Source: CAD feature listing. Evaluate the final solid. Frame: model axes, mm. Give positions to 0.01 mm unless a question says otherwise; leave off trailing zeros. Write each loop counter-clockwise with the first axis right and the second up, starting at its lowest first coordinate (ties: lowest second). Pieces come first, ordered by that corner, then holes. Notation, with made-up numbers: M -20,62 L 36,62 A29 cw 36,96 Z; hole C 82,-35.5 d7. An arc over 180 degrees is marked long. Return JSON: item names as keys, results as strings.
```python
from build123d import *

# Parameters (mm, degrees)
PARED_Y_1_4IN_START          = 95.25
CROQUIS1_W                   = 228.6
CROQUIS1_H                   = 50.8
PARED_Y_1_4IN_DEPTH          = 6.35
ROSCA_M3_INFERIOR_START      = 12.7
CROQUIS2_R                   = 1.25
ROSCA_M3_INFERIOR_DEPTH      = 10
ROSCA_M3_SUPERIOR_START      = 53.5
CROQUIS3_R                   = 1.25
ROSCA_M3_SUPERIOR_DEPTH      = 10
BARRENOS_M3_ESQUINAS_START   = 95.25
CROQUIS4_R                   = 1.7
BARRENOS_M3_ESQUINAS_DEPTH   = 6.35
REFRENTADO_M3_ESQUINAS_START = 98.4
CROQUIS5_R                   = 2.9
REFRENTADO_M3_ESQUINAS_DEPTH = 3.2
RANURAS_VENTILACION_START    = 95.25
RANURAS_VENTILACION_DEPTH    = 6.35


with BuildPart() as part:
    # Croquis1 → Pared_+Y_1-4in (new body)
    with BuildSketch(Plane(origin=(0, 0, 0), x_dir=(1, 0, 0), z_dir=(0, 1, 0)).offset(PARED_Y_1_4IN_START)):
        with Locations((-25.4, -38.1)):
            Rectangle(CROQUIS1_W, CROQUIS1_H)
    extrude(amount=PARED_Y_1_4IN_DEPTH)

    # Croquis2 → Rosca_M3_inferior (cut)
    with BuildSketch(Plane.XY.offset(ROSCA_M3_INFERIOR_START)):
        with Locations((-125, 98.425)):
            Circle(CROQUIS2_R)
        with Locations((-30, 98.425)):
            Circle(CROQUIS2_R)
        with Locations((70, 98.425)):
            Circle(CROQUIS2_R)
    extrude(amount=ROSCA_M3_INFERIOR_DEPTH, mode=Mode.SUBTRACT)

    # Croquis3 → Rosca_M3_superior (cut)
    with BuildSketch(Plane.XY.offset(ROSCA_M3_SUPERIOR_START)):
        with Locations((-125, 98.425)):
            Circle(CROQUIS3_R)
        with Locations((-30, 98.425)):
            Circle(CROQUIS3_R)
        with Locations((70, 98.425)):
            Circle(CROQUIS3_R)
    extrude(amount=ROSCA_M3_SUPERIOR_DEPTH, mode=Mode.SUBTRACT)

    # Croquis4 → Barrenos_M3_esquinas (cut)
    with BuildSketch(Plane(origin=(0, 0, 0), x_dir=(1, 0, 0), z_dir=(0, 1, 0)).offset(BARRENOS_M3_ESQUINAS_START)):
        with Locations(Location((-136.525, -25, 0), (0, 0, 270))):
            Circle(CROQUIS4_R)
        with Locations(Location((-136.525, -50, 0), (0, 0, 270))):
            Circle(CROQUIS4_R)
        with Locations(Location((85.725, -25, 0), (0, 0, 270))):
            Circle(CROQUIS4_R)
        with Locations(Location((85.725, -50, 0), (0, 0, 270))):
            Circle(CROQUIS4_R)
    extrude(amount=BARRENOS_M3_ESQUINAS_DEPTH, mode=Mode.SUBTRACT)

    # Croquis5 → Refrentado_M3_esquinas (cut)
    with BuildSketch(Plane(origin=(0, 0, 0), x_dir=(1, 0, 0), z_dir=(0, 1, 0)).offset(REFRENTADO_M3_ESQUINAS_START)):
        with Locations(Location((-136.525, -25, 0), (0, 0, 270))):
            Circle(CROQUIS5_R)
        with Locations(Location((-136.525, -50, 0), (0, 0, 270))):
            Circle(CROQUIS5_R)
        with Locations(Location((85.725, -25, 0), (0, 0, 270))):
            Circle(CROQUIS5_R)
        with Locations(Location((85.725, -50, 0), (0, 0, 270))):
            Circle(CROQUIS5_R)
    extrude(amount=REFRENTADO_M3_ESQUINAS_DEPTH, mode=Mode.SUBTRACT)

    # Croquis6 → Ranuras_ventilacion (cut)
    with BuildSketch(Plane(origin=(0, 0, 0), x_dir=(1, 0, 0), z_dir=(0, 1, 0)).offset(RANURAS_VENTILACION_START)):
        with BuildLine():
            Line((-107, -24.7), (-107, -51.5))
            ThreePointArc((-107, -51.5), (-110, -54.5), (-113, -51.5))
            Line((-113, -51.5), (-113, -24.7))
            ThreePointArc((-113, -24.7), (-110, -21.7), (-107, -24.7))
        make_face()
        with BuildLine():
            Line((-92, -24.7), (-92, -51.5))
            ThreePointArc((-92, -51.5), (-95, -54.5), (-98, -51.5))
            Line((-98, -51.5), (-98, -24.7))
            ThreePointArc((-98, -24.7), (-95, -21.7), (-92, -24.7))
        make_face()
        with BuildLine():
            Line((-77, -24.7), (-77, -51.5))
            ThreePointArc((-77, -51.5), (-80, -54.5), (-83, -51.5))
            Line((-83, -51.5), (-83, -24.7))
            ThreePointArc((-83, -24.7), (-80, -21.7), (-77, -24.7))
        make_face()
        with BuildLine():
            Line((-62, -24.7), (-62, -51.5))
            ThreePointArc((-62, -51.5), (-65, -54.5), (-68, -51.5))
            Line((-68, -51.5), (-68, -24.7))
            ThreePointArc((-68, -24.7), (-65, -21.7), (-62, -24.7))
        make_face()
        with BuildLine():
            Line((-42, -24.7), (-42, -51.5))
            ThreePointArc((-42, -51.5), (-45, -54.5), (-48, -51.5))
            Line((-48, -51.5), (-48, -24.7))
            ThreePointArc((-48, -24.7), (-45, -21.7), (-42, -24.7))
        make_face()
        with BuildLine():
            Line((-12, -24.7), (-12, -51.5))
            ThreePointArc((-12, -51.5), (-15, -54.5), (-18, -51.5))
            Line((-18, -51.5), (-18, -24.7))
            ThreePointArc((-18, -24.7), (-15, -21.7), (-12, -24.7))
        make_face()
        with BuildLine():
            Line((3, -24.7), (3, -51.5))
            ThreePointArc((3, -51.5), (0, -54.5), (-3, -51.5))
            Line((-3, -51.5), (-3, -24.7))
            ThreePointArc((-3, -24.7), (0, -21.7), (3, -24.7))
        make_face()
        with BuildLine():
            Line((18, -24.7), (18, -51.5))
            ThreePointArc((18, -51.5), (15, -54.5), (12, -51.5))
            Line((12, -51.5), (12, -24.7))
            ThreePointArc((12, -24.7), (15, -21.7), (18, -24.7))
        make_face()
        with BuildLine():
            Line((33, -24.7), (33, -51.5))
            ThreePointArc((33, -51.5), (30, -54.5), (27, -51.5))
            Line((27, -51.5), (27, -24.7))
            ThreePointArc((27, -24.7), (30, -21.7), (33, -24.7))
        make_face()
        with BuildLine():
            Line((48, -24.7), (48, -51.5))
            ThreePointArc((48, -51.5), (45, -54.5), (42, -51.5))
            Line((42, -51.5), (42, -24.7))
            ThreePointArc((42, -24.7), (45, -21.7), (48, -24.7))
        make_face()
        with BuildLine():
            Line((58, -24.7), (58, -51.5))
            ThreePointArc((58, -51.5), (55, -54.5), (52, -51.5))
            Line((52, -51.5), (52, -24.7))
            ThreePointArc((52, -24.7), (55, -21.7), (58, -24.7))
        make_face()
    extrude(amount=RANURAS_VENTILACION_DEPTH, mode=Mode.SUBTRACT)


solid = part.part
```
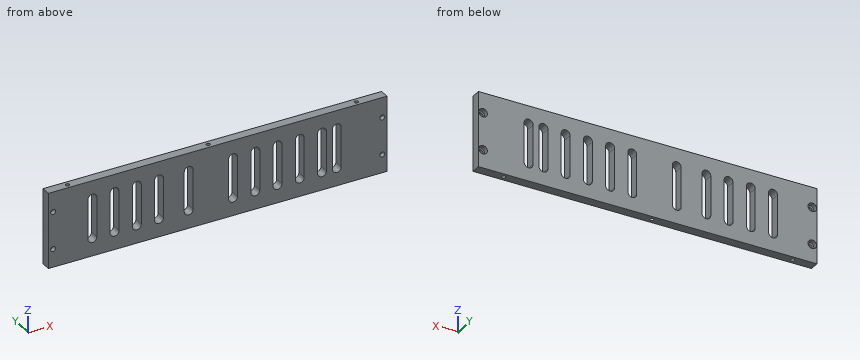
1) Cut plane A-A, the plane x = 0. Return the cut outline in (y, z).
Numbers:
{"outline": "M 95.25,12.7 L 101.6,12.7 L 101.6,21.7 L 95.25,21.7 Z; M 95.25,54.5 L 101.6,54.5 L 101.6,63.5 L 95.25,63.5 Z"}
2) Line query: line 1 (X direction, y = 98.5, z = 15.5); line 2 (Z direction, x = -78, y = 97.75); line 3 (Z direction, x = -64, y = 99.25). Output: solid intervals per line, ascending. Write a range as [from, to].
Numbers:
{"line 1": "x = [-139.7, -126.25], [-123.75, -31.25], [-28.75, 68.75], [71.25, 88.9]", "line 2": "z = [12.7, 22.46], [53.74, 63.5]", "line 3": "z = [12.7, 21.87], [54.33, 63.5]"}
3) Cut plane B-B, the plane x = -66. Return the cut outline in (y, z), then the cut area to 3 significant figures.
Numbers:
{"outline": "M 95.25,12.7 L 101.6,12.7 L 101.6,21.87 L 95.25,21.87 Z; M 95.25,54.33 L 101.6,54.33 L 101.6,63.5 L 95.25,63.5 Z", "area": "116 mm²"}
4) Contact query for a flat-ended pin moving along its axis: pin 1 Ø5 at (x, z) = (-136.525, 50) entering from +Y. Output: stop coordinate, or through.
Numbers:
{"pin 1": "stops at y = 98.4"}
